```python
from build123d import *

# Parameters (mm, degrees)
SKETCH1_W           = 500
SKETCH1_H           = 200
BOSS_EXTRUDE1_DEPTH = 10
FILLET1_R           = 50
SKETCH2_R           = 4
SKETCH2_R_2         = 2
CUT_EXTRUDE2_DEPTH  = 10


with BuildPart() as part:
    # Sketch1 → Boss-Extrude1 (new body)
    with BuildSketch(Plane(origin=(0, 0, 0), x_dir=(1, 0, 0), z_dir=(0, 1, 0))):
        with Locations((250, 100)):
            Rectangle(SKETCH1_W, SKETCH1_H)
    extrude(amount=BOSS_EXTRUDE1_DEPTH)

    # Fillet1
    fillet1_edges = [part.edges().sort_by_distance(p)[0] for p in [
        (0, 5, -200),
        (500, 5, -200),
        (500, 5, 0),
        (0, 5, 0),
    ]]
    fillet(fillet1_edges, radius=FILLET1_R)

    # Sketch2 → Cut-Extrude2 (cut)
    with BuildSketch(Plane(origin=(0, 10, 0), x_dir=(1, 0, 0), z_dir=(0, 1, 0))):
        with Locations(Location((42, 41.5, 0), (0, 0, 270))):
            Circle(SKETCH2_R)
        with Locations(Location((42, 158.5, 0), (0, 0, 270))):
            Circle(SKETCH2_R)
        with Locations(Location((108.274847281, 70.5, 0), (0, 0, 270))):
            Circle(SKETCH2_R_2)
        with Locations(Location((133.274847281, 70.5, 0), (0, 0, 270))):
            Circle(SKETCH2_R_2)
        with Locations(Location((158.274847281, 70.5, 0), (0, 0, 270))):
            Circle(SKETCH2_R_2)
        with Locations(Location((183.274847281, 70.5, 0), (0, 0, 270))):
            Circle(SKETCH2_R_2)
        with Locations(Location((208.274847281, 70.5, 0), (0, 0, 270))):
            Circle(SKETCH2_R_2)
        with Locations(Location((233.274847281, 70.5, 0), (0, 0, 270))):
            Circle(SKETCH2_R_2)
        with Locations(Location((258.274847281, 70.5, 0), (0, 0, 270))):
            Circle(SKETCH2_R_2)
        with Locations(Location((283.274847281, 70.5, 0), (0, 0, 270))):
            Circle(SKETCH2_R_2)
        with Locations(Location((308.274847281, 70.5, 0), (0, 0, 270))):
            Circle(SKETCH2_R_2)
        with Locations(Location((333.274847281, 70.5, 0), (0, 0, 270))):
            Circle(SKETCH2_R_2)
        with Locations(Location((358.274847281, 70.5, 0), (0, 0, 270))):
            Circle(SKETCH2_R_2)
        with Locations(Location((383.274847281, 70.5, 0), (0, 0, 270))):
            Circle(SKETCH2_R_2)
        with Locations(Location((133.274847281, 129.5, 0), (0, 0, 270))):
            Circle(SKETCH2_R_2)
        with Locations(Location((158.274847281, 129.5, 0), (0, 0, 270))):
            Circle(SKETCH2_R_2)
        with Locations(Location((180.998972497, 129.5, 0), (0, 0, 270))):
            Circle(SKETCH2_R_2)
        with Locations(Location((208.274847281, 129.5, 0), (0, 0, 270))):
            Circle(SKETCH2_R_2)
        with Locations(Location((233.274847281, 129.5, 0), (0, 0, 270))):
            Circle(SKETCH2_R_2)
        with Locations(Location((258.274847281, 129.5, 0), (0, 0, 270))):
            Circle(SKETCH2_R_2)
        with Locations(Location((283.274847281, 129.5, 0), (0, 0, 270))):
            Circle(SKETCH2_R_2)
        with Locations(Location((308.274847281, 129.5, 0), (0, 0, 270))):
            Circle(SKETCH2_R_2)
        with Locations(Location((333.274847281, 129.5, 0), (0, 0, 270))):
            Circle(SKETCH2_R_2)
        with Locations(Location((358.274847281, 129.5, 0), (0, 0, 270))):
            Circle(SKETCH2_R_2)
        with Locations(Location((383.274847281, 129.5, 0), (0, 0, 270))):
            Circle(SKETCH2_R_2)
        with Locations(Location((108.274847281, 129.5, 0), (0, 0, 270))):
            Circle(SKETCH2_R_2)
        with Locations(Location((40, 115, 0), (0, 0, 270))):
            Circle(SKETCH2_R_2)
        with Locations(Location((65, 115, 0), (0, 0, 270))):
            Circle(SKETCH2_R_2)
        with Locations(Location((65, 85, 0), (0, 0, 270))):
            Circle(SKETCH2_R_2)
        with Locations(Location((40, 85, 0), (0, 0, 270))):
            Circle(SKETCH2_R_2)
        with BuildLine():
            Line((105, 115), (405, 115))
            ThreePointArc((405, 115), (420, 100), (405, 85))
            Line((405, 85), (105, 85))
            ThreePointArc((105, 85), (90, 100), (105, 115))
        make_face()
        with BuildLine():
            Line((427, 138.5), (452, 138.5))
            ThreePointArc((452, 138.5), (456.5, 134), (452, 129.5))
            Line((452, 129.5), (427, 129.5))
            ThreePointArc((427, 129.5), (422.5, 134), (427, 138.5))
        make_face()
        with BuildLine():
            Line((427, 70.5), (452, 70.5))
            ThreePointArc((452, 70.5), (456.5, 66), (452, 61.5))
            Line((452, 61.5), (427, 61.5))
            ThreePointArc((427, 61.5), (422.5, 66), (427, 70.5))
        make_face()
        with BuildLine():
            Line((108.274847281, 160), (198.274847281, 160))
            ThreePointArc((198.274847281, 160), (205.774847281, 167.5), (198.274847281, 175))
            Line((198.274847281, 175), (108.274847281, 175))
            ThreePointArc((108.274847281, 175), (100.774847281, 167.5), (108.274847281, 160))
        make_face()
        with BuildLine():
            Line((278.274847281, 160), (370, 160))
            ThreePointArc((370, 160), (377.5, 167.5), (370, 175))
            Line((370, 175), (278.274847281, 175))
            ThreePointArc((278.274847281, 175), (270.774847281, 167.5), (278.274847281, 160))
        make_face()
        with BuildLine():
            Line((110, 25), (200, 25))
            ThreePointArc((200, 25), (207.5, 32.5), (200, 40))
            Line((200, 40), (110, 40))
            ThreePointArc((110, 40), (102.5, 32.5), (110, 25))
        make_face()
        with BuildLine():
            Line((280, 25), (370, 25))
            ThreePointArc((370, 25), (377.5, 32.5), (370, 40))
            Line((370, 40), (280, 40))
            ThreePointArc((280, 40), (272.5, 32.5), (280, 25))
        make_face()
    extrude(amount=-CUT_EXTRUDE2_DEPTH, mode=Mode.SUBTRACT)


solid = part.part
```
Verification items for the finished model (mm, model axes). A direction names the side the tool comes from. Give positions to 0.01 mm unless a question says otherwise; leave off trailing zeros. Order: outer loops, then holes, each group sorted by start corner. A loop starts at its lowest first (then second) coordinate and runs counter-clockwise, first axis right, second up. Notation, with made-up numbers: (66, 50.25) -> (123, 50.25) arc R13 ccw to (123, 72.25) -> close; hole circle Ø3 at (89.5, -34.75). An arc over 180 degrees is marked (long way). Use a Markdown table: item, result.
1) Depth check by flat-ended pin: pin 1 Ø2.5 at (x, z) = (383.27, -70.5) entering from +Y. Enter the tip coordinate at first touch or a pass-through.
Results:
| item | result |
|---|---|
| pin 1 | through |
2) Section check A-A, the plane x = 340. Record the boundary of the cut face in (y, z).
Results:
| item | result |
|---|---|
| outline | (0, -200) -> (10, -200) -> (10, -175) -> (0, -175) -> close; (0, -160) -> (10, -160) -> (10, -115) -> (0, -115) -> close; (0, -85) -> (10, -85) -> (10, -40) -> (0, -40) -> close; (0, -25) -> (10, -25) -> (10, 0) -> (0, 0) -> close |
3) Section check C-C, the plane z = -92. Record the boundary of the cut face in (x, y), then the cut area to 3 significant figures.
Results:
| item | result |
|---|---|
| outline | (0, 0) -> (92.31, 0) -> (92.31, 10) -> (0, 10) -> close; (417.69, 0) -> (500, 0) -> (500, 10) -> (417.69, 10) -> close |
| area | 1,750 mm² |
4) Mould release check, pull along Z, two halves, no side actions. Record for faces 3 (the flat face through (154, 5, -25)), 4 (the flat face through (247, 5, 0)), 5 (the flat face through (247, 10, -124)): pulls with the +Z half, pulls with the -Z half, needs draft (parallel to the pull), parting line crosses it, or undercut.
Results:
| item | result |
|---|---|
| face 3 | undercut |
| face 4 | pulls with the +Z half |
| face 5 | needs draft |
5) Material ranges on probe 1 along Z at (x, y) = (165.5, 4.25); probe 2 along Z at (x, y) = (248, 7); probe 3 along X at (y, z) = (5.5, -173.5), recorded low to high.
Results:
| item | result |
|---|---|
| probe 1 | -200 to -175, -160 to -115, -85 to -40, -25 to 0 |
| probe 2 | -200 to -115, -85 to 0 |
| probe 3 | 5.87 to 103.77, 202.77 to 273.77, 374.5 to 494.13 |
6) Section check D-D, the plane z = -167.5. Record the boundary of the cut face in (x, y), then the cut area to 3 significant figures.
Results:
| item | result |
|---|---|
| outline | (3.16, 0) -> (100.77, 0) -> (100.77, 10) -> (3.16, 10) -> close; (205.77, 0) -> (270.77, 0) -> (270.77, 10) -> (205.77, 10) -> close; (377.5, 0) -> (496.84, 0) -> (496.84, 10) -> (377.5, 10) -> close |
| area | 2,820 mm² |
7) Tool access check on faces 1 (the cylindrical face through (377.5, 5.07, -167.34)), 2 (the cylindrical face through (484.964, 5.07, -14.258)). Record the directions out of +Z, -Z, +X, -X, +Y, -Y that give a thin tool (end or side, any length) a straight path to the whole face; none if there is none.
Results:
| item | result |
|---|---|
| face 1 | +Y, -Y |
| face 2 | +Z, +X, +Y, -Y |
8) Section check B-B, the plane z = -32.5. Record the boundary of the cut face in (x, y), then the cut area to 3 significant figures.
Results:
| item | result |
|---|---|
| outline | (3.16, 0) -> (102.5, 0) -> (102.5, 10) -> (3.16, 10) -> close; (207.5, 0) -> (272.5, 0) -> (272.5, 10) -> (207.5, 10) -> close; (377.5, 0) -> (496.84, 0) -> (496.84, 10) -> (377.5, 10) -> close |
| area | 2,840 mm² |
